Read the model definition and answer for the solid it produces. Units are mm, in the model's axes. Face numbers are marked on the shaded views. A direction names the side the tool comes from. Give positions to 0.01 mm unless a question says otherwise; leave off trailing zeros. Order: outer loops, then holes, each group sorted by start corner. A loop starts at its lowest first (then second) coordinate and runs counter-clockwise, first axis right, second up.
Autodesk Inventor part; units mm, degrees
ref_plane "YZ Plane" through (0, 0, 0) normal (1, 0, 0) x (0, 1, 0)
ref_plane "XZ Plane" through (0, 0, 0) normal (0, 1, 0) x (-1, 0, 0)
ref_plane "XY Plane" through (0, 0, 0) normal (0, 0, 1) x (1, 0, 0)
sketch "Skizze1" plane through (0, 0, 0) normal (0, 1, 0) x (-1, 0, 0)
  line L0 (0, 0) -> (60, 0)
  line L1 (60, 0) -> (60, -120)
  line L2 (60, -120) -> (0, -120)
  line L3 (0, -120) -> (0, 0)
  dimension "d0" = 120
  dimension "d1" = 60
extrude "Extrusion1" add sketch "Skizze1" along normal blind 5
sketch "Skizze2" plane through (0, 5, 0) normal (0, 1, 0) x (1, 0, 0)
  circle A0 centre (-30, 10) radius 4.9
  circle A1 centre (-30, 40) radius 4.9
  circle A2 centre (-30, 90) radius 4.9
  line L0 (-60, 0) -> (0, 0)
  line L1 (0, 0) -> (0, 120)
  dimension "d4" = 10
  dimension "d5" = 30
  dimension "d6" = 50
  dimension "d7" = 30
  dimension "d8" = 30
  dimension "d9" = 30
  dimension "d10" = 9.8
  dimension "d11" = 9.8
  dimension "d12" = 9.8
extrude "Extrusion2" add sketch "Skizze2" along normal blind 20
sketch "Skizze3" plane through (0, 0, -120) normal (0, 0, -1) x (-1, 0, 0)
  line L0 (25.1, 5) -> (25.1, 25)
  line L1 (25.1, 6.7142) -> (25.1, 25)
  line L2 (34.9, 5) -> (34.9, 25)
  line L3 (34.9, 5) -> (34.9, 25)
  line L4 (60, 5) -> (0, 5)
  line L5 (23.3172, 25) -> (26.1, 25)
  line L6 (26.1, 25) -> (26.1, 17)
  line L7 (26.1, 17) -> (23.3172, 17)
  line L8 (23.3172, 17) -> (23.3172, 25)
  line L9 (36.4895, 25) -> (33.9, 25)
  line L10 (33.9, 25) -> (33.9, 17)
  line L11 (33.9, 17) -> (36.4895, 17)
  line L12 (36.4895, 17) -> (36.4895, 25)
  line L13 (34.9, 25) -> (25.1, 25)
  point P0 (0, 0)
  dimension "d19" = 8
  dimension "d20" = 1
  dimension "d21" = 1
extrude "Extrusion3" cut sketch "Skizze3" against normal blind 120 contours L7 L8 L5 L0 | L0 L5 L6 L7 | L11 L10 L9 L2 | L2 L9 L12 L11
sketch "Skizze4" plane through (0, 5, 0) normal (0, 1, 0) x (1, 0, 0)
  line L0 (0, 0) -> (0, 120)
  line L1 (-60, 0) -> (0, 0)
  line L2 (-60, 120) -> (-60, 0)
  line L3 (0, 120) -> (-60, 120)
  point P0 (-8, 8)
  point P1 (-52, 8)
  point P2 (-8, 112)
  point P3 (-52, 112)
  dimension "d31" = 8
  dimension "d32" = 8
  dimension "d33" = 8
  dimension "d34" = 8
  dimension "d35" = 8
  dimension "d36" = 8
  dimension "d37" = 8
  dimension "d38" = 8
  dimension "d39" = 104
  dimension "d40" = 44
hole "Bohrung1" at (-8, 5, -8) at (-52, 5, -8) at (-8, 5, -112) at (-52, 5, -112) direction (0, -1, 0) diameter 4 depth 5
properties part number "Gear_Platte_3D-Druck_3D-Druck"
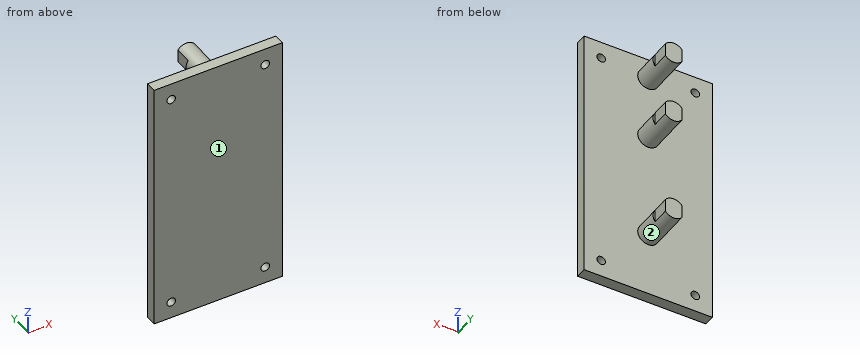
1) Given pin 1 (1.1 mm diameter, centred on x = -34.5, z = -11.5, fed in from +Y); pin 2 (4.5 mm diameter, centred on y = 22, z = -9.5, fed in from +X); pin 3 (10 mm diameter, centred on y = 12.5, z = -40, fed in from +X), each flat-ended and moving along its own axis, determine where each tip first touches the part or whether it passes through.
Final values:
pin 1: stops at y = 17
pin 2: stops at x = -26.1
pin 3: stops at x = -25.1
2) A tool of negligible diameter and unlimited length cuts with its end or side. For the marked faces 1 and 2, from which of +Z, -Z, +X, -X, +Y, -Y can it reach the whole face along a straight path? Write none if from no direction.
Final values:
face 1: +Z, -Z, +X, -X, -Y
face 2: +Y
3) Consider L1, parallel to X at y = 2.3, z = -112; L2, parallel to Z at x = -52, y = 3.5; L3, parallel to Y at x = -15.5, z = -88. Determine where each line is inside the solid, lowest interval first.
Final values:
L1: x = -60 to -54, -50 to -10, -6 to 0
L2: z = -120 to -114, -110 to -10, -6 to 0
L3: y = 0 to 5
4) The part is cut by section D-D on x = -45. Determine the outline of the cut face in (y, z), and give its area (3 significant figures).
Final values:
outline: (0, -120) - (5, -120) - (5, 0) - (0, 0) - close
area: 600 mm2
5) The part is cut by section C-C on z = -40. Determine the outline of the cut face in (x, y).
Final values:
outline: (-60, 0) - (0, 0) - (0, 5) - (-25.1, 5) - (-25.1, 17) - (-26.1, 17) - (-26.1, 25) - (-33.9, 25) - (-33.9, 17) - (-34.9, 17) - (-34.9, 5) - (-60, 5) - close
6) The part is cut by section B-B on x = -52. Determine the outline of the cut face in (y, z).
Final values:
outline: (0, -120) - (5, -120) - (5, -114) - (0, -114) - close; (0, -110) - (5, -110) - (5, -10) - (0, -10) - close; (0, -6) - (5, -6) - (5, 0) - (0, 0) - close
7) The part is cut by section A-A on y = 18.25. Determine the outline of the cut face in (x, z), and give its area (3 significant figures).
Final values:
outline: (-33.9, -92.97) arc R4.9 ccw to (-26.1, -92.97) - (-26.1, -87.03) arc R4.9 ccw to (-33.9, -87.03) - close; (-33.9, -42.97) arc R4.9 ccw to (-26.1, -42.97) - (-26.1, -37.03) arc R4.9 ccw to (-33.9, -37.03) - close; (-33.9, -12.97) arc R4.9 ccw to (-26.1, -12.97) - (-26.1, -7.03) arc R4.9 ccw to (-33.9, -7.03) - close
area: 202 mm2
